Can you work these out from the model? Positions are in its coordinate system, mm. A direction names the side the tool comes from. Coordinates: 2 decimals unless noted, no trailing zeros. Order: outer loops, then holes, each group sorted by start corner. A loop starts at its lowest first (then second) coordinate and runs counter-clockwise, first axis right, second up. Notation, with made-up numbers: (64.5, 59.25) -> (76.5, 59.25) arc R23 ccw to (76.5, 83.25) -> close; hole circle Ø10 at (85.5, -35.75). An arc over 180 degrees is marked (long way). Answer in a Markdown table with one row per item.
```python
from build123d import *

# Parameters (mm, degrees)
SKETCH4_R               = 5
CUT_EXTRUDE2_DEPTH      = 440.0500001
CUT_EXTRUDE2_DEPTH_BACK = 20.0500001


with BuildPart() as part:
    # Sweep-Thin1: sweep along a path in Sketch1
    with BuildLine(Plane(origin=(0, 0, 0), x_dir=(1, 0, 0), z_dir=(0, 1, 0))) as sweep_thin1_path:
        Line((0, 0), (0, 810))
        ThreePointArc((0, 810), (11.715728753, 838.284271247), (40, 850))
        Line((40, 850), (380, 850))
        ThreePointArc((380, 850), (408.284271247, 838.284271247), (420, 810))
        Line((420, 810), (420, 0))
    # Sketch3 → Sweep-Thin1 (sweep)
    with BuildSketch(Plane.XY):
        with BuildLine():
            Line((14.05, 19.05), (-14.05, 19.05))
            ThreePointArc((-14.05, 19.05), (-17.585533906, 17.585533906), (-19.05, 14.05))
            Line((-19.05, 14.05), (-19.05, -14.05))
            ThreePointArc((-19.05, -14.05), (-17.585533906, -17.585533906), (-14.05, -19.05))
            Line((-14.05, -19.05), (14.05, -19.05))
            ThreePointArc((14.05, -19.05), (17.585533906, -17.585533906), (19.05, -14.05))
            Line((19.05, -14.05), (19.05, 14.05))
            ThreePointArc((19.05, 14.05), (17.585533906, 17.585533906), (14.05, 19.05))
        make_face()
        with BuildLine():
            Line((14.05, 15.875), (-14.05, 15.875))
            ThreePointArc((-14.05, 15.875), (-15.340469876, 15.340469876), (-15.875, 14.05))
            Line((-15.875, 14.05), (-15.875, -14.05))
            ThreePointArc((-15.875, -14.05), (-15.340469876, -15.340469876), (-14.05, -15.875))
            Line((-14.05, -15.875), (14.05, -15.875))
            ThreePointArc((14.05, -15.875), (15.340469876, -15.340469876), (15.875, -14.05))
            Line((15.875, -14.05), (15.875, 14.05))
            ThreePointArc((15.875, 14.05), (15.340469876, 15.340469876), (14.05, 15.875))
        make_face(mode=Mode.SUBTRACT)
    sweep(path=sweep_thin1_path.line)

    # Sketch4 → Cut-Extrude2 (cut, two sides)
    with BuildSketch(Plane(origin=(0, 0, 0), x_dir=(0, 0, -1), z_dir=(1, 0, 0))) as cut_extrude2_sk:
        with Locations((30, 0)):
            Circle(SKETCH4_R)
        with Locations((80, 0)):
            Circle(SKETCH4_R)
        with Locations((180.955115779, 0)):
            Circle(SKETCH4_R)
    extrude(amount=CUT_EXTRUDE2_DEPTH, mode=Mode.SUBTRACT)
    extrude(cut_extrude2_sk.sketch, amount=-CUT_EXTRUDE2_DEPTH_BACK, mode=Mode.SUBTRACT)


solid = part.part
```
(1) I need wall thicknesses on line 1 (X direction, y = -3, z = -401) (3 decimals); line 2 (Z direction, x = 196, y = 14) (3 decimals). Which ranges of each line are inside material? Lowest first, please. Write a range as [from, to].
Response values:
| item | result |
|---|---|
| line 1 | [-19.05, -15.875], [15.875, 19.05], [400.95, 404.125], [435.875, 439.05] |
| line 2 | [-869.05, -865.875], [-834.125, -830.95] |
(2) Will these pins go through, and if not, where does the flat tip stop? pin 1 Ø8 at (y, z) = (0, -30) entering from -X; pin 2 Ø5 at (x, y) = (354.5, 8.5) entering from +Z.
Response values:
| item | result |
|---|---|
| pin 1 | through |
| pin 2 | z = -830.95 |
(3) We'd pull the mould along X, two halves only. Please class faces 1 (the flat face through (400.95, 0, -399)), 2 (the flat face through (-15.875, 0, -411)), 3 (the flat face through (439.05, 0, -399)), 4 (the flat face through (-19.05, 0, -411)): +X half, -X half, draft (parallel to the pull), parting line (faces both ways), or undercut.
Response values:
| item | result |
|---|---|
| face 1 | undercut |
| face 2 | undercut |
| face 3 | +X half |
| face 4 | -X half |
(4) On a 3-axis mill with a long thin cutter (end or side, diameter ignored), from which of +Z, -Z, +X, -X, +Y, -Y can I reach the whole of each face in a straight line? I mean faces 5 (the cylindrical face through (421.293, -0.197, -852.211)), 6 (the flat face through (410, 19.05, -498)), 7 (the cylindrical face through (22.755, -0.197, -826.87)), 8 (the flat face through (404.125, 0, -399)), 9 (the flat face through (212, 0, -830.95)). Say none if no direction works.
Response values:
| item | result |
|---|---|
| face 5 | -Z, +X, +Y, -Y |
| face 6 | +Z, -Z, +X, -X, +Y |
| face 7 | none |
| face 8 | +Z |
| face 9 | +Z, +Y, -Y |
(5) Suppose I cut it at B-B (x = 368). Please give me the cut outline in (y, z) (3 decimals).
Response values:
| item | result |
|---|---|
| outline | (-19.05, -864.05) arc R5 ccw to (-14.05, -869.05) -> (14.05, -869.05) arc R5 ccw to (19.05, -864.05) -> (19.05, -835.95) arc R5 ccw to (14.05, -830.95) -> (-14.05, -830.95) arc R5 ccw to (-19.05, -835.95) -> close; hole (-15.875, -864.05) arc R1.825 ccw to (-14.05, -865.875) -> (14.05, -865.875) arc R1.825 ccw to (15.875, -864.05) -> (15.875, -835.95) arc R1.825 ccw to (14.05, -834.125) -> (-14.05, -834.125) arc R1.825 ccw to (-15.875, -835.95) -> close |
(6) Suppose I cut it at A-A (z = -387.5). Count the separate pieces of the cut face and the enclosed holes in it, and give its area (3 significant figures).
Response values:
| item | result |
|---|---|
| separate pieces | 2 |
| enclosed holes | 2 |
| area | 850 mm2 |
